from build123d import *

# Parameters (mm, degrees)
SKETCH002_W     = 103
SKETCH002_H     = 30
PAD002_DEPTH    = 9
SKETCH003_R     = 12.5
SKETCH003_W     = 38
SKETCH003_H     = 26
POCKET_DEPTH    = 7
SKETCH004_W     = 103
SKETCH004_H     = 30
SKETCH004_W_2   = 101
SKETCH004_H_2   = 28
POCKET001_DEPTH = 3
SKETCH007_W     = 3.602402
SKETCH007_H     = 11.897104
POCKET003_DEPTH = 10


with BuildPart() as part:
    # Sketch002 → Pad002 (new body)
    with BuildSketch(Plane.XY):
        Rectangle(SKETCH002_W, SKETCH002_H)
    extrude(amount=PAD002_DEPTH)

    # Sketch003 (on Pad) → Pocket (cut)
    with BuildSketch(Plane.XY.offset(2)):
        with Locations((37, 0)):
            Circle(SKETCH003_R)
        with Locations((-30.5, 0)):
            Rectangle(SKETCH003_W, SKETCH003_H)
        with BuildLine():
            ThreePointArc((12.562178, 9.129165), (6.5, 12.629165), (0.437822, 9.129165))
            Line((-6.062178, -2.129165), (0.437822, 9.129165))
            ThreePointArc((-6.062178, -2.129165), (-6.062178, -9.129165), (0, -12.629165))
            Line((13, -12.629165), (0, -12.629165))
            ThreePointArc((13, -12.629165), (19.062178, -9.129165), (19.062178, -2.129165))
            Line((12.562178, 9.129165), (19.062178, -2.129165))
        make_face()
    extrude(amount=POCKET_DEPTH, mode=Mode.SUBTRACT)

    # Sketch004 (on Face5 of Pocket) → Pocket001 (cut)
    with BuildSketch(Plane.XY.offset(9)):
        Rectangle(SKETCH004_W, SKETCH004_H)
        Rectangle(SKETCH004_W_2, SKETCH004_H_2, mode=Mode.SUBTRACT)
    extrude(amount=-POCKET001_DEPTH, mode=Mode.SUBTRACT)

    # Sketch007 (on Face11 of Pocket001) → Pocket003 (cut)
    with BuildSketch(Plane.XY.offset(9)):
        with Locations((49.698799, 0)):
            Rectangle(SKETCH007_W, SKETCH007_H)
    extrude(amount=-POCKET003_DEPTH, mode=Mode.SUBTRACT)


solid = part.part
Verification items for the finished model (mm, model axes). A direction names the side the tool comes from. Coordinates: 2 decimals unless noted, no trailing zeros. Order: outer loops, then holes, each group sorted by start corner. A loop starts at its lowest first (then second) coordinate and runs counter-clockwise, first axis right, second up.
Item 1: Depth check by flat-ended pin: pin 1 (5 mm diameter, centred on x = -24, y = -9, fed in from -Z); pin 2 (1.5 mm diameter, centred on x = 18.5, z = 7, fed in from +Y); pin 3 (1.6 mm diameter, centred on y = 0.5, z = 1, fed in from +X); pin 4 (1.5 mm diameter, centred on y = -10, z = 8, fed in from +X). Enter the tip coordinate at first touch or a pass-through.
Filled in:
pin 1: stops at z = 0
pin 2: stops at y = 14
pin 3: stops at x = 47.9
pin 4: stops at x = 50.5
Item 2: Material ranges on L1, parallel to X at y = 0, z = 4; L2, parallel to X at y = -0.75, z = 3.25; L3, parallel to X at y = 9.5, z = 5.5, recorded low to high.
Filled in:
L1: x = -51.5 to -49.5, -11.5 to -4.83, 17.83 to 24.5
L2: x = -51.5 to -49.5, -11.5 to -5.27, 18.27 to 24.52
L3: x = -51.5 to -49.5, -11.5 to 0.67, 12.33 to 28.88, 45.12 to 51.5
Item 3: Access from +Z, -Z, +X, -X, +Y, -Y to the whole of each face (thin tool, end or side, straight path). Record for faces 4 (the face through (-50.5, 0, 8)), 5 (the face through (-1, -14, 8)), 6 (the face through (-31, 13, 5)).
Filled in:
face 4: +Z, -X, +Y, -Y
face 5: +Z, +X, -X, -Y
face 6: +Z
Item 4: Section check B-B, the plane x = 37. Enter the section's corners in (y, z).
Filled in:
outline: (-15, 0) - (15, 0) - (15, 6) - (14, 6) - (14, 9) - (12.5, 9) - (12.5, 2) - (-12.5, 2) - (-12.5, 9) - (-14, 9) - (-14, 6) - (-15, 6) - close
Item 5: Release check for a two-part mould opening along X. For faces 1 (the face through (-0.2, 14.5, 6)), 2 (the face through (50.5, -10, 8)), 3 (the face through (-2.86, 3.42, 5.45)) record: +X half, -X half, draft (parallel to the pull), parting line (faces both ways), or undercut.
Filled in:
face 1: draft
face 2: +X half
face 3: undercut
Item 6: Section check C-C, the plane y = -10.25. Enter the section's corners in (x, z), then the cut area to 3 significant figures.
Filled in:
outline: (-51.5, 0) - (51.5, 0) - (51.5, 6) - (50.5, 6) - (50.5, 9) - (44.15, 9) - (44.15, 2) - (29.85, 2) - (29.85, 9) - (18.26, 9) - (18.26, 2) - (-5.26, 2) - (-5.26, 9) - (-11.5, 9) - (-11.5, 2) - (-49.5, 2) - (-49.5, 9) - (-50.5, 9) - (-50.5, 6) - (-51.5, 6) - close
area: 390 mm2
Item 7: Section check D-D, the plane x = -9. Enter the section's corners in (y, z).
Filled in:
outline: (-15, 0) - (15, 0) - (15, 6) - (14, 6) - (14, 9) - (-14, 9) - (-14, 6) - (-15, 6) - close
Item 8: Section check A-A, the plane z = 7. Enter the section's corners in (x, y).
Filled in:
outline: (-50.5, -14) - (50.5, -14) - (50.5, -5.95) - (47.99, -5.95) arc R12.5 cw (long way) to (47.99, 5.95) - (50.5, 5.95) - (50.5, 14) - (-50.5, 14) - close; hole (-49.5, -13) - (-11.5, -13) - (-11.5, 13) - (-49.5, 13) - close; hole (-6.06, -2.13) arc R7 ccw to (0, -12.63) - (13, -12.63) arc R7 ccw to (19.06, -2.13) - (12.56, 9.13) arc R7 ccw to (0.44, 9.13) - close
